Here's how the part is built. I have some questions about the finished solid (model axes, mm). A direction names the side the tool comes from. Round coordinates to 2 decimals unless told otherwise and drop trailing zeros. Write each loop counter-clockwise with the first axis right and the second up, starting at its lowest first coordinate (ties: lowest second). Pieces come first, ordered by that corner, then holes. Notation, with made-up numbers: (39.25, -21) -> (89.25, -21) arc R21 ccw to (89.25, -14) -> close; hole circle Ø10 at (6.5, 84). An arc over 180 degrees is marked (long way). Answer in a Markdown table with one row per item.
from build123d import *
from build123d.topology import SkipClean

# Parameters (mm, degrees)
SKETCH1_R            = 150
BOSS_EXTRUDE1_DEPTH  = 200
BOSS_EXTRUDE11_DEPTH = 300
BOSS_EXTRUDE14_START = -300
SKETCH12_R           = 125
BOSS_EXTRUDE14_DEPTH = 400
SKETCH13_W           = 400
SKETCH13_H           = 350
SKETCH13_R           = 10
BOSS_EXTRUDE15_DEPTH = 50
SKETCH13_3_W         = 46.677917496
SKETCH13_3_H         = 80
SKETCH13_3_R         = 10
SKETCH13_3_W_2       = 50
BOSS_EXTRUDE16_DEPTH = 20
BOSS_EXTRUDE17_DEPTH = 90
SKETCH16_R           = 25
BOSS_EXTRUDE18_DEPTH = 150
FILLET2_R            = 10
FILLET3_R            = 20


with BuildPart() as part:
    # Sketch1 → Boss-Extrude1 (new body)
    with BuildSketch(Plane.XY):
        Circle(SKETCH1_R)
    extrude(amount=BOSS_EXTRUDE1_DEPTH)

    # Sketch7 → Boss-Extrude11 (add)
    with SkipClean():  # the faces are left unmerged after this step: merging them gives an invalid solid
        with BuildSketch(Plane.XY.offset(200)):
            with BuildLine():
                Line((-90, 120), (90, 120))
                ThreePointArc((90, 120), (101.396020382, 110.538893837), (111.803398875, 100))
                Line((111.803398875, 100), (-111.803398875, 100))
                ThreePointArc((-111.803398875, 100), (-101.396020382, 110.538893837), (-90, 120))
            make_face()
            with BuildLine():
                Line((-126.885775404, 80), (126.885775404, 80))
                ThreePointArc((126.885775404, 80), (132.559251115, 70.200035213), (137.477270849, 60))
                Line((137.477270849, 60), (-137.477270849, 60))
                ThreePointArc((-137.477270849, 60), (-132.559251115, 70.200035213), (-126.885775404, 80))
            make_face()
            with BuildLine():
                Line((144.16342013, -41.435592144), (-144.16342013, -41.435592144))
                ThreePointArc((-144.16342013, -41.435592144), (-146.803816882, -30.799989431), (-148.660687473, -20))
                Line((-148.660687473, -20), (148.660687473, -20))
                ThreePointArc((148.660687473, -20), (146.803816882, -30.799989431), (144.16342013, -41.435592144))
            make_face()
            with BuildLine():
                Line((111.803398875, -100), (-111.803398875, -100))
                ThreePointArc((-111.803398875, -100), (-101.396020382, -110.538893837), (-90, -120))
                Line((-90, -120), (90, -120))
                ThreePointArc((90, -120), (101.396020382, -110.538893837), (111.803398875, -100))
            make_face()
            with BuildLine():
                Line((144.568322948, 40), (-144.568322948, 40))
                ThreePointArc((-144.568322948, 40), (-146.955139883, 30.069700063), (-148.660687473, 20))
                Line((-148.660687473, 20), (148.660687473, 20))
                ThreePointArc((148.660687473, 20), (146.955139883, 30.069700063), (144.568322948, 40))
            make_face()
            with BuildLine():
                Line((137.477270849, -60), (-137.477270849, -60))
                ThreePointArc((-137.477270849, -60), (-133.599215205, -68.20007109), (-129.232599216, -76.150740639))
                Line((-129.232599216, -76.150740639), (129.232599216, -76.150740639))
                ThreePointArc((129.232599216, -76.150740639), (133.599215205, -68.20007109), (137.477270849, -60))
            make_face()
        extrude(amount=BOSS_EXTRUDE11_DEPTH)



with BuildPart() as body_2:
    # Sketch12 → Boss-Extrude14 (new body)
    with BuildSketch(Plane.XY.offset(500).offset(BOSS_EXTRUDE14_START)):
        Circle(SKETCH12_R)
    extrude(amount=BOSS_EXTRUDE14_DEPTH)


with BuildPart() as body_3:
    # Sketch13 → Boss-Extrude15 (new body)
    with BuildSketch(Plane(origin=(0, -220, 0), x_dir=(-1, 0, 0), z_dir=(0, -1, 0))):
        with Locations((0, -274.735715433)):
            Rectangle(SKETCH13_W, SKETCH13_H)
        with Locations(Location((-175, -139.735715433, 0), (0, 0, 180))):
            Circle(SKETCH13_R, mode=Mode.SUBTRACT)
        with Locations(Location((-175, -409.735715433, 0), (0, 0, 180))):
            Circle(SKETCH13_R, mode=Mode.SUBTRACT)
        with Locations(Location((175, -409.735715433, 0), (0, 0, 180))):
            Circle(SKETCH13_R, mode=Mode.SUBTRACT)
        with Locations(Location((175, -139.735715433, 0), (0, 0, 180))):
            Circle(SKETCH13_R, mode=Mode.SUBTRACT)
    extrude(amount=-BOSS_EXTRUDE15_DEPTH)

    # Sketch13<3> → Boss-Extrude16 (add)
    # profile 1 of 4: a face of its own
    with BuildSketch(Plane(origin=(0, -220, 0), x_dir=(-1, 0, 0), z_dir=(0, -1, 0))):
        with Locations((-176.661041252, -409.735715433)):
            Rectangle(SKETCH13_3_W, SKETCH13_3_H)
        with Locations(Location((-175, -409.735715433, 0), (0, 0, 180))):
            Circle(SKETCH13_3_R, mode=Mode.SUBTRACT)
    # profile 2 of 4: a face of its own
    with BuildSketch(Plane(origin=(0, -220, 0), x_dir=(-1, 0, 0), z_dir=(0, -1, 0))):
        with Locations((-176.661041252, -139.735715433)):
            Rectangle(SKETCH13_3_W, SKETCH13_3_H)
        with Locations(Location((-175, -139.735715433, 0), (0, 0, 180))):
            Circle(SKETCH13_3_R, mode=Mode.SUBTRACT)
    # profile 3 of 4: a face of its own
    with BuildSketch(Plane(origin=(0, -220, 0), x_dir=(-1, 0, 0), z_dir=(0, -1, 0))):
        with Locations((175, -409.735715433)):
            Rectangle(SKETCH13_3_W_2, SKETCH13_3_H)
        with Locations(Location((175, -409.735715433, 0), (0, 0, 180))):
            Circle(SKETCH13_3_R, mode=Mode.SUBTRACT)
    # profile 4 of 4: a face of its own
    with BuildSketch(Plane(origin=(0, -220, 0), x_dir=(-1, 0, 0), z_dir=(0, -1, 0))):
        with Locations((175, -139.735715433)):
            Rectangle(SKETCH13_3_W_2, SKETCH13_3_H)
        with Locations(Location((175, -139.735715433, 0), (0, 0, 180))):
            Circle(SKETCH13_3_R, mode=Mode.SUBTRACT)
    extrude(amount=BOSS_EXTRUDE16_DEPTH)


with BuildPart() as part_1:
    with SkipClean():  # the faces are left unmerged after this step: merging them gives an invalid solid
        add(part.part)

        add(body_2.part)  # Boss-Extrude17 merges body 2

        add(body_3.part)  # Boss-Extrude17 merges body 3
        # Sketch14 → Boss-Extrude17 (add, symmetric)
        with BuildSketch(Plane.XY.offset(274.735715433)):
            Polygon((-200, -170), (200, -170), (100, -110), (-100, -110), align=None)
        extrude(amount=BOSS_EXTRUDE17_DEPTH, both=True)

    # Sketch16 → Boss-Extrude18 (add)
    with BuildSketch(Plane.XY.offset(600)):
        Circle(SKETCH16_R)
    extrude(amount=BOSS_EXTRUDE18_DEPTH)

    # Fillet2
    fillet2_edges = [part_1.edges().sort_by_distance(p)[0] for p in [
        (-25, 0, 600),
    ]]
    fillet(fillet2_edges, radius=FILLET2_R)

    # Fillet3
    fillet3_edges = [part_1.edges().sort_by_distance(p)[0] for p in [
        (-125, 0, 600),
        (-150, 0, 0),
    ]]
    fillet(fillet3_edges, radius=FILLET3_R)


solid = part_1.part
1) Which directions (+Z, -Z, +X, -X, +Y, -Y) give clear straight access to the entire face, cutting with the end or side of a thin tool? Please do faces 1 (the face through (-131, -41.436, 348)), 2 (the face through (3, -198, 99.736)), 3 (the face through (-133, -31, 500)), 4 (the face through (-134, 30, 500)).
Response:
| item | result |
|---|---|
| face 1 | +Z, -X |
| face 2 | -Z, +X, -X, -Y |
| face 3 | +Z, -X, -Y |
| face 4 | +Z, -X, +Y |
2) I want a section at A-A, the plane x = 0. List the corners of the cut face in (y, z) for me.
Response:
| item | result |
|---|---|
| outline | (-220, 99.74) -> (-170, 99.74) -> (-170, 184.74) -> (-150, 184.74) -> (-150, 20) arc R20 ccw to (-130, 0) -> (130, 0) arc R20 ccw to (150, 20) -> (150, 200) -> (125, 200) -> (125, 580) arc R20 ccw to (105, 600) -> (35, 600) arc R10 cw to (25, 610) -> (25, 750) -> (-25, 750) -> (-25, 610) arc R10 cw to (-35, 600) -> (-105, 600) arc R20 ccw to (-125, 580) -> (-125, 364.74) -> (-170, 364.74) -> (-170, 449.74) -> (-220, 449.74) -> close |
3) We'd pull the mould along X, two halves only. Please class faces 5 (the face through (3, -170, 407)), 6 (the face through (179.61, -204.51, 400.86)), 7 (the face through (-200, -198, 277)), 8 (the face through (151.291, -140.775, 275.996)): +X half, -X half, draft (parallel to the pull), parting line (faces both ways), or undercut.
Response:
| item | result |
|---|---|
| face 5 | draft |
| face 6 | undercut |
| face 7 | -X half |
| face 8 | +X half |
4) I want a section at C-C, the plane y = 0. List the corners of the cut face in (x, z) for me.
Response:
| item | result |
|---|---|
| outline | (-150, 20) arc R20 ccw to (-130, 0) -> (130, 0) arc R20 ccw to (150, 20) -> (150, 200) -> (125, 200) -> (125, 580) arc R20 ccw to (105, 600) -> (35, 600) arc R10 cw to (25, 610) -> (25, 750) -> (-25, 750) -> (-25, 610) arc R10 cw to (-35, 600) -> (-105, 600) arc R20 ccw to (-125, 580) -> (-125, 200) -> (-150, 200) -> close |
5) I need wall thicknesses on line 1 (Z direction, x = -175, y = -191); line 2 (Z direction, x = -175, y = -233); line 3 (Y direction, x = 77, z = 321). Which ranges of each line are inside material? Lowest first, please. Write a range as [from, to].
Response:
| item | result |
|---|---|
| line 1 | z = [99.74, 129.74], [149.74, 399.74], [419.74, 449.74] |
| line 2 | z = [99.74, 129.74], [149.74, 179.74], [369.74, 399.74], [419.74, 449.74] |
| line 3 | y = [-220, -100], [-98.47, 98.47], [100, 120] |
6) I want a section at B-B, the plane x = -175. List the corners of the cut face in (y, z) for me, and give its area (3 significant figures).
Response:
| item | result |
|---|---|
| outline | (-240, 99.74) -> (-170, 99.74) -> (-170, 129.74) -> (-240, 129.74) -> close; (-240, 149.74) -> (-170, 149.74) -> (-170, 184.74) -> (-155, 184.74) -> (-155, 364.74) -> (-170, 364.74) -> (-170, 399.74) -> (-240, 399.74) -> (-240, 369.74) -> (-220, 369.74) -> (-220, 179.74) -> (-240, 179.74) -> close; (-240, 419.74) -> (-170, 419.74) -> (-170, 449.74) -> (-240, 449.74) -> close |
| area | 20,600 mm^2 |
7) For pin 1 (3 mm diameter, centred on x = -70.5, z = 507, fed in from +Y); pin 2 (16 mm diameter, centred on x = -184.5, y = -233, fed in from +Z); pin 3 (10 mm diameter, centred on x = 74, z = 274.5, fed in from +Y); pin 4 (4 mm diameter, centred on x = -42, y = -62.5, fed in from -Z), each with a flat end and sliding along its axis, tell me the tip position at first contact or that it passes through.
Response:
| item | result |
|---|---|
| pin 1 | stops at y = 104.23 |
| pin 2 | stops at z = 449.74 |
| pin 3 | stops at y = 120 |
| pin 4 | stops at z = 0 |
8) I want a section at D-D, the plane z = 556. List the corners of the cut face in (x, y) for me, and give its area (3 significant figures).
Response:
| item | result |
|---|---|
| outline | circle Ø250 at (0, 0) |
| area | 49,100 mm^2 |
